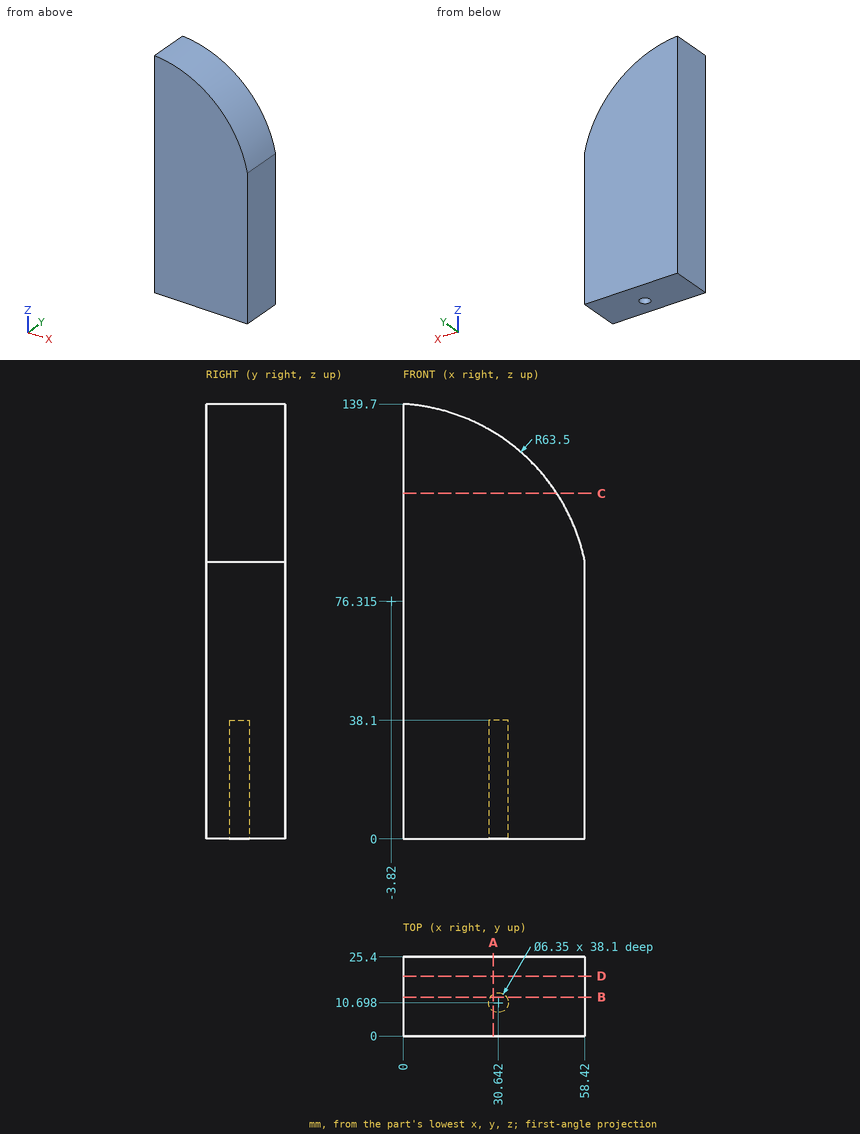
Here's the drawing with two shaded views (mm, measured from the low corner). I have some questions. Round coordinates to 2 decimals unless told otherwise and drop trailing zeros. Loops run counter-clockwise (first coordinate to the right, second up) from the corner with the lowest first, then second, coordinate; pieces in that order, holes last.
Item 1: Suppose I cut it at D-D, the plane y = 19.25. Write out the boundary of the cut face in (x, z) (1 decimal).
Item 2: Suppose I cut it at A-A, the plane x = 29. Write out the boundary of the cut face in (y, z) (1 decimal).
Item 3: Please list where these lines run through material, in increasing order: L1, parallel to X at y = 4.5, z = 133 (1 decimal); L2, parallel to X at y = 13.75, z = 114.5 (1 decimal); L3, parallel to Z at x = 19.5, y = 9.25.
Item 4: Will these pins go through, and if not, where does the flat tip stop? pin 1 Ø10 at (x, y) = (16.5, 9) entering from -Z; pin 2 Ø7.5 at (x, y) = (30.64, 10.7) entering from +Z (1 decimal).
Item 5: Suppose I cut it at B-B, the plane y = 12.5. Write out the boundary of the cut face in (x, z) (1 decimal).
Item 6: Suppose I cut it at C-C, the plane z = 111. Write out the boundary of the cut face in (x, y).
Reported:
1. outline: (0, 0) - (58.4, 0) - (58.4, 88.9) arc R63.5 ccw to (0, 139.7) - close
2. outline: (0, 0) - (8, 0) - (8, 38.1) - (13.4, 38.1) - (13.4, 0) - (25.4, 0) - (25.4, 130.7) - (0, 130.7) - close
3. L1: x = 0 to 24.8
3. L2: x = 0 to 46.9
3. L3: z = 0 to 135.38
4. pin 1: stops at z = 0
4. pin 2: stops at z = 131.9
5. outline: (0, 0) - (28, 0) - (28, 38.1) - (33.3, 38.1) - (33.3, 0) - (58.4, 0) - (58.4, 88.9) arc R63.5 ccw to (0, 139.7) - close
6. outline: (0, 0) - (49.37, 0) - (49.37, 25.4) - (0, 25.4) - close
